Geometry: see drawing. Coordinates: mm, zero at the bounding-box minimum. A direction names the side the tool comes from. Coordinates: 2 decimals unless noted, no trailing zeros. Loops run counter-clockwise (first coordinate to the right, second up) from the corner with the lowest first, then second, coordinate; pieces in that order, holes last. Notation, with made-up numbers: (44.5, 61.5) - (83.5, 61.5) arc R8 cw to (83.5, 69.5) - close; hole circle Ø11 at (-5, 25.5). An arc over 180 degrees is marked (long way). Answer in a Markdown table with one row per item.
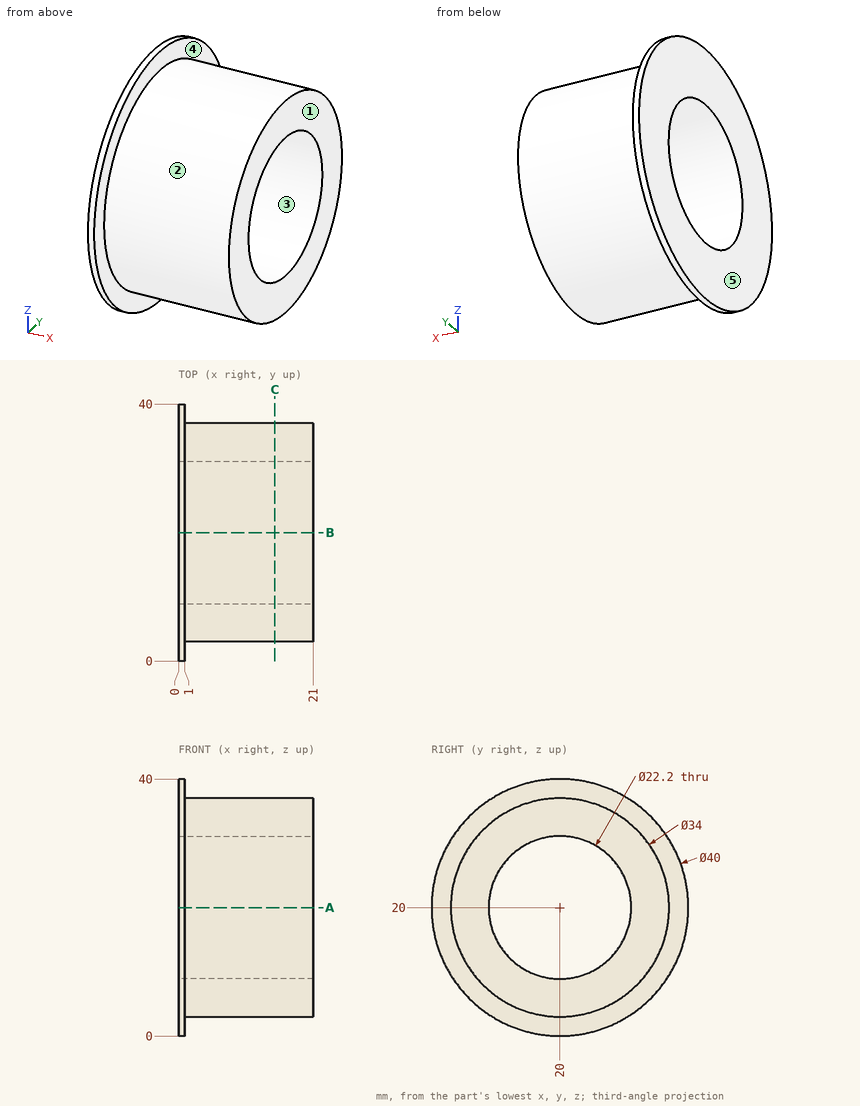
(1) First-contact query: pin 1 Ø1 at (x, z) = (7, 30.5) entering from -Y; pin 2 Ø2 at (x, z) = (5.5, 35.5) entering from +Y; pin 3 Ø3 at (x, z) = (18.5, 14) entering from +Y. Flat tips, straight axial feed; report the tip coordinate or a pass-through.
Verdict:
| item | result |
|---|---|
| pin 1 | stops at y = 6.25 |
| pin 2 | stops at y = 28.87 |
| pin 3 | stops at y = 36.39 |
(2) Cut plane A-A on z = 20. Output: boundary loops of the cut face in (x, y), then the cut area to 3 significant figures.
Verdict:
| item | result |
|---|---|
| outline | (0, 0) - (1, 0) - (1, 3) - (21, 3) - (21, 8.9) - (0, 8.9) - close; (0, 31.1) - (21, 31.1) - (21, 37) - (1, 37) - (1, 40) - (0, 40) - close |
| area | 254 mm² |
(3) Pull-direction query (Y, two-part tool) for the marked faces 1, 2 and 3; classes: pulls with the +Y half, pulls with the -Y half, needs draft (parallel to the pull), parting line crosses it, or undercut.
Verdict:
| item | result |
|---|---|
| face 1 | needs draft |
| face 2 | parting line crosses it |
| face 3 | undercut |
(4) Ray query, probe 1 along Y at (x, z) = (15.5, 20); probe 2 along X at (y, z) = (20, 2.5); probe 3 along Z at (x, y) = (7.25, 18). Return the intervals inside material, ascending.
Verdict:
| item | result |
|---|---|
| probe 1 | y = 3 to 8.9, 31.1 to 37 |
| probe 2 | x = 0 to 1 |
| probe 3 | z = 3.12 to 9.08, 30.92 to 36.88 |
(5) Access query for the marked faces 4 and 5. Directions: +Z, -Z, +X, -X, +Y, -Y. A direction counts if a zero-diameter tool reaches every point of the face in a straight line with its end or side. Return the directions, or none.
Verdict:
| item | result |
|---|---|
| face 4 | +X |
| face 5 | +Z, -Z, -X, +Y, -Y |
(6) Cut plane C-C on x = 15. Output: boundary loops of the cut face in (y, z), then the cut area to 3 significant figures.
Verdict:
| item | result |
|---|---|
| outline | circle Ø34 at (20, 20); hole circle Ø22.2 at (20, 20) |
| area | 521 mm² |
